Source: CAD feature listing. Evaluate the final solid. Frame: model axes, mm. Face numbers are marked on the shaded views. A direction names the side the tool comes from. Coordinates: 2 decimals unless noted, no trailing zeros. Write each loop counter-clockwise with the first axis right and the second up, starting at its lowest first coordinate (ties: lowest second). Pieces come first, ordered by that corner, then holes. Notation, with made-up numbers: M 84,0.25 L 116,0.25 A22 cw 116,30.25 Z; hole C 25,69.25 d7. An arc over 180 degrees is marked long. One line per item, written item: value. Start each with the question number.
Item 1: Set-up query: the marked faces 1, 2 and 3. Return all of +Z, -Z, +X, -X, +Y, -Y with unobstructed straight access to the full face (end or side cutting, diameter ignored); none if empty.
Item 2: Cut plane D-D, the plane z = 8.75. Output: boundary loops of the cut face in (x, y).
Item 3: Pin query (flat end, axial travel): P1, Ø4, axis at x = -11, z = 24, coming from the -Y side; P2, Ø4, axis at y = 11.5, z = 9.5, coming from the -X side; P3, Ø5, axis at x = 0, y = 11, coming from the +Z side; P4, Ø6.5, axis at x = 11.5, z = 18, coming from the +Y side. Return the tip coordinate at first contact, or that it passes through.
Item 4: Cut plane C-C, the plane x = 0. Output: boundary loops of the cut face in (y, z).
Item 5: Cut plane B-B, the plane z = 24. Output: boundary loops of the cut face in (x, y).
Item 6: Mould query, pull axis X, two halves, no side actions, for the marked faces 4, 5 and 6. Classes: released by +X, released by -X, zero draft, split by the parting line, or undercut.
Item 7: Cut plane A-A, the plane y = 11. Output: boundary loops of the cut face in (x, z), then the cut area to 3 significant figures.
Item 8: Ray query, L1, parallel to X at y = 5.25, z = 6; L2, parallel to Z at x = 13, y = 12.5; L3, parallel to X at y = 15.5, z = 7.5. Return the intervals inside material, ascending. Write a range as from..to.
```python
from build123d import *

# Parameters (mm, degrees)
SKETCH_1_R          = 4
EXTRUDE_1_DEPTH     = 30
SKETCH_3_R          = 2
CUT_EXTRUDE_1_DEPTH = 41.902322672


with BuildPart() as part:
    # 草图1 → 凸台-拉伸1 (new body)
    with BuildSketch(Plane.XY):
        Polygon((17, 0), (-17, 0), (-17, 6), (-15.5, 7.5), (-15.5, 18), (-9.5, 18), (-5.5, 22), (5.5, 22), (9.5, 18), (15.5, 18), (15.5, 7.5), (17, 6), align=None)
        with Locations((0, 11)):
            Circle(SKETCH_1_R, mode=Mode.SUBTRACT)
    extrude(amount=EXTRUDE_1_DEPTH)

    # 草图3 → 切除-拉伸1 (cut, through all)
    with BuildSketch(Plane.XZ):
        with Locations(Location((12, 24, 0), (0, 0, 270))):
            Circle(SKETCH_3_R)
        with Locations(Location((-12, 24, 0), (0, 0, 270))):
            Circle(SKETCH_3_R)
        with Locations(Location((-12, 6, 0), (0, 0, 270))):
            Circle(SKETCH_3_R)
        with Locations(Location((12, 6, 0), (0, 0, 270))):
            Circle(SKETCH_3_R)
    extrude(amount=-CUT_EXTRUDE_1_DEPTH, mode=Mode.SUBTRACT)


solid = part.part
```
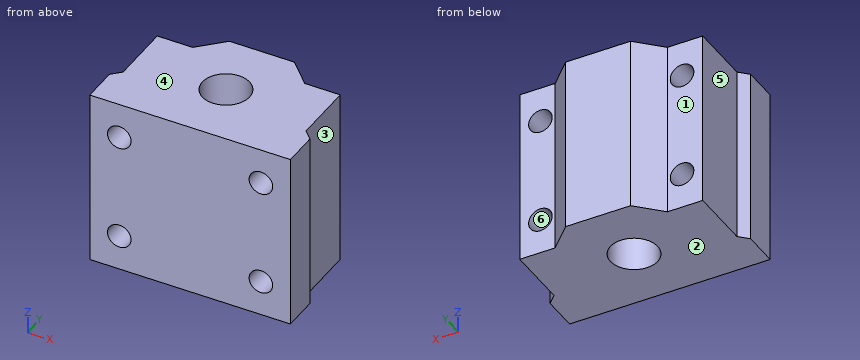
From the geometry:
1. face 1: +Z, -Z, -X, +Y
1. face 2: -Z, +X, -X, +Y, -Y
1. face 3: +Z, -Z, +X, +Y
2. outline: M -17,0 L 17,0 L 17,6 L 15.5,7.5 L 15.5,18 L 9.5,18 L 5.5,22 L -5.5,22 L -9.5,18 L -15.5,18 L -15.5,7.5 L -17,6 Z; hole C 0,11 d8
3. P1: stops at y = 0
3. P2: stops at x = -15.5
3. P3: passes through
3. P4: stops at y = 19.25
4. outline: M 0,0 L 7,0 L 7,30 L 0,30 Z; M 15,0 L 22,0 L 22,30 L 15,30 Z
5. outline: M -17,0 L -14,0 L -14,18 L -15.5,18 L -15.5,7.5 L -17,6 Z; M -10,0 L 10,0 L 10,18 L 9.5,18 L 5.5,22 L -5.5,22 L -9.5,18 L -10,18 Z; M 14,0 L 17,0 L 17,6 L 15.5,7.5 L 15.5,18 L 14,18 Z; hole C 0,11 d8
6. face 4: zero draft
6. face 5: released by -X
6. face 6: undercut
7. outline: M -15.5,0 L -4,0 L -4,30 L -15.5,30 Z; M 4,0 L 15.5,0 L 15.5,30 L 4,30 Z; hole C -12,6 d4; hole C -12,24 d4; hole C 12,6 d4; hole C 12,24 d4
7. area: 640 mm²
8. L1: x = -17..-14, -10..10, 14..17
8. L2: z = 0..4.27, 7.73..22.27, 25.73..30
8. L3: x = -15.5..-13.32, -10.68..10.68, 13.32..15.5
